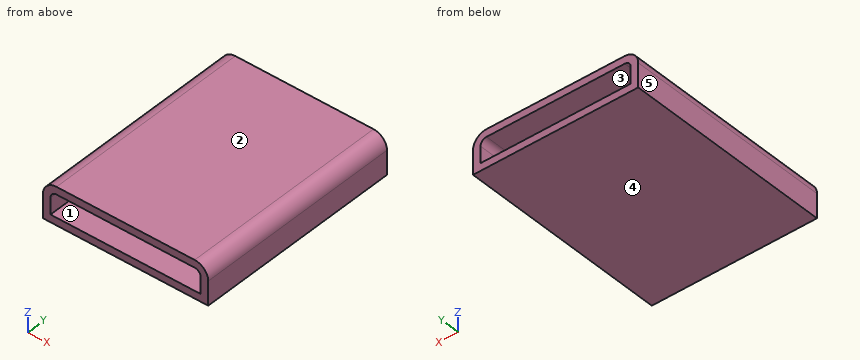
from build123d import *

# Parameters (mm, degrees)
BOSS_EXTRUDE1_DEPTH = 88.9
CUT_EXTRUDE1_DEPTH  = 88.9


with BuildPart() as part:
    # Sketch1 → Boss-Extrude1 (new body)
    with BuildSketch(Plane(origin=(0, 0, 0), x_dir=(1, 0, 0), z_dir=(0, 1, 0))):
        with BuildLine():
            Line((-3.175, 6.985), (-3.175, 2.54))
            ThreePointArc((-3.175, 2.54), (-1.501115254, -1.501115254), (2.54, -3.175))
            Line((2.54, -3.175), (60.96, -3.175))
            ThreePointArc((60.96, -3.175), (65.001115254, -1.501115254), (66.675, 2.54))
            Line((66.675, 2.54), (66.675, 6.985))
            Line((66.675, 6.985), (66.675, 12.7))
            Line((66.675, 12.7), (60.96, 12.7))
            Line((60.96, 12.7), (2.54, 12.7))
            Line((2.54, 12.7), (-3.175, 12.7))
            Line((-3.175, 12.7), (-3.175, 6.985))
        make_face()
    extrude(amount=BOSS_EXTRUDE1_DEPTH)

    # Sketch2 → Cut-Extrude1 (cut)
    with BuildSketch(Plane(origin=(0, 88.9, 0), x_dir=(1, 0, 0), z_dir=(0, 1, 0))):
        with BuildLine():
            Line((2.54, 9.525), (0, 9.525))
            Line((0, 9.525), (0, 6.985))
            Line((0, 6.985), (0, 2.54))
            ThreePointArc((0, 2.54), (0.743948776, 0.743948776), (2.54, 0))
            Line((2.54, 0), (60.96, 0))
            ThreePointArc((60.96, 0), (62.756051224, 0.743948776), (63.5, 2.54))
            Line((63.5, 2.54), (63.5, 6.985))
            Line((63.5, 6.985), (63.5, 9.525))
            Line((63.5, 9.525), (60.96, 9.525))
            Line((60.96, 9.525), (2.54, 9.525))
        make_face()
    extrude(amount=-CUT_EXTRUDE1_DEPTH, mode=Mode.SUBTRACT)


solid = part.part
Source: CAD feature listing. Evaluate the final solid. Frame: model axes, mm. Face numbers are marked on the shaded views. A direction names the side the tool comes from. Round coordinates to 2 decimals unless told otherwise and drop trailing zeros. Loops run counter-clockwise (first coordinate to the right, second up) from the corner with the lowest first, then second, coordinate; pieces in that order, holes last. Notation, with made-up numbers: (-15, -6) - (-1, -6) arc R29 cw to (-1, 32) - close; hole circle Ø9 at (25.5, 47.5). An arc over 180 degrees is marked (long way). Write item = value, one per line. Start each with the question number.
(1) Ray query, line 1 along Z through (x, y) = (13.5, 39) (3 decimals); line 2 along X through (y, z) = (60, -2.25); line 3 along X through (y, z) = (29.5, -0.75). Return the intervals inside material, ascending. Write a range as from..to.
(2) Section query B-B, the plane z = -6.25. Output: boundary loops of the cut face in (x, y) (3 decimals), plus the area to 3 significant figures.
(3) Pull-direction query (X, two-part tool) for the marked faces 3, 4 and 5; classes: +X half, -X half, draft (parallel to the pull), parting line (faces both ways), or undercut.
(4) Pin query (flat end, axial travel): pin 1 (6 mm diameter, centred on y = 79, z = -1.5, fed in from +X) (3 decimals); pin 2 (3 mm diameter, centred on y = 31.5, z = -0.5, fed in from -X). Return the tip coordinate at first contact, or that it passes through.
(5) Section query A-A, the plane x = 14. Output: boundary loops of the cut face in (y, z) (3 decimals).
(6) Section query C-C, the plane y = 10. Output: boundary loops of the cut face in (x, z) (3 decimals), plus the area to 3 significant figures.
(7) Set-up query: the marked faces 1 and 2. Return all of +Z, -Z, +X, -X, +Y, -Y with unobstructed straight access to the full face (end or side cutting, diameter ignored); none if empty.
Conclusion:
q1.line_1 = -12.7..-9.525, 0..3.175
q1.line_2 = -3.17..0.02, 63.48..66.67
q1.line_3 = -2.89..0.74, 62.76..66.39
q2.outline = (-3.175, 0) - (0, 0) - (0, 88.9) - (-3.175, 88.9) - close; (63.5, 0) - (66.675, 0) - (66.675, 88.9) - (63.5, 88.9) - close
q2.area = 565 mm2
q3.face_3 = undercut
q3.face_4 = draft
q3.face_5 = -X half
q4.pin_1 = 66.675
q4.pin_2 = -3.15
q5.outline = (0, -12.7) - (88.9, -12.7) - (88.9, -9.525) - (0, -9.525) - close; (0, 0) - (88.9, 0) - (88.9, 3.175) - (0, 3.175) - close
q6.outline = (-3.175, -12.7) - (66.675, -12.7) - (66.675, -2.54) arc R5.715 ccw to (60.96, 3.175) - (2.54, 3.175) arc R5.715 ccw to (-3.175, -2.54) - close; hole (0, -9.525) - (63.5, -9.525) - (63.5, -2.54) arc R2.54 ccw to (60.96, 0) - (2.54, 0) arc R2.54 ccw to (0, -2.54) - close
q6.area = 493 mm2
q7.face_1 = +Y, -Y
q7.face_2 = +Z, +X, -X, +Y, -Y
